For this review, take the finished solid that the model builds, in its own axes (mm). Coordinates: 2 decimals unless noted, no trailing zeros. Loops run counter-clockwise (first coordinate to the right, second up) from the corner with the lowest first, then second, coordinate; pieces in that order, holes last.
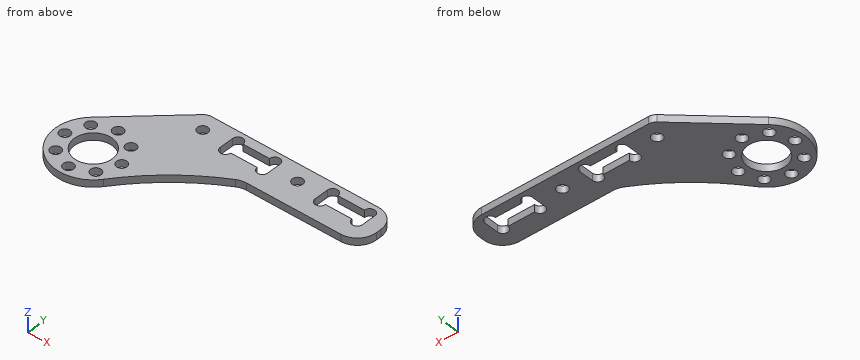
Autodesk Inventor part; units mm, degrees
ref_plane "YZ Plane" through (0, 0, 0) normal (1, 0, 0) x (0, 1, 0)
ref_plane "XZ Plane" through (0, 0, 0) normal (0, 1, 0) x (-1, 0, 0)
ref_plane "XY Plane" through (0, 0, 0) normal (0, 0, 1) x (1, 0, 0)
sketch "スケッチ1" plane through (0, 0, 0) normal (0, 0, 1) x (1, 0, 0)
  circle A0 centre (8.8, 8.8) radius 8
  circle A1 centre (2.8, 8.8) radius 0.825
  circle A2 centre (4.5574, 4.5574) radius 0.825
  circle A3 centre (8.8, 2.8) radius 0.825
  circle A4 centre (13.0426, 4.5574) radius 0.825
  circle A5 centre (14.8, 8.8) radius 0.825
  circle A6 centre (13.0426, 13.0426) radius 0.825
  circle A7 centre (8.8, 14.8) radius 0.825
  circle A8 centre (4.5574, 13.0426) radius 0.825
  circle A9 centre (8.8, 8.8) radius 4
  circle A10 centre (8.8, 14.8) radius 1.1
  circle A11 centre (4.5574, 13.0426) radius 1.1
  circle A12 centre (2.8, 8.8) radius 1.1
  circle A13 centre (4.5574, 4.5574) radius 1.1
  circle A14 centre (8.8, 2.8) radius 1.1
  circle A15 centre (13.0426, 4.5574) radius 1.1
  circle A16 centre (14.8, 8.8) radius 1.1
  circle A17 centre (13.0426, 13.0426) radius 1.1
  line L0 (3.3206, 14.6289) -> (16.8, 27.3)
  line L1 (23.8, 25.3) -> (33.8, 25.3)
  line L2 (33.8, 25.3) -> (33.8, 22.3)
  line L3 (33.8, 22.3) -> (23.8, 22.3)
  line L4 (23.8, 22.3) -> (23.8, 25.3)
  circle A18 centre (24.9, 25.3) radius 1.1
  line L5 (28.8, 25.3) -> (28.8, 22.3) construction
  line L6 (28.8, 23.8) -> (23.8, 23.8) construction
  circle A19 centre (24.9, 22.3) radius 1.1
  circle A20 centre (32.7, 25.3) radius 1.1
  circle A21 centre (32.7, 22.3) radius 1.1
  circle A22 centre (38.8, 23.8) radius 1.1
  circle A23 centre (18.8, 23.8) radius 1.1
  line L7 (16.8, 27.3) -> (40.8, 27.3)
  line L8 (40.8, 27.3) -> (40.8, 21.8)
  arc A24 (40.8, 21.8) -> (15.1891, 3.9855) centre (55.1209, -26.1052) ccw
  point P0 (0, 0)
  point P1 (31.6, 22.3)
  point P2 (26, 22.3)
  point P3 (26, 25.3)
  point P4 (31.6, 25.3)
  dimension "d7" = 2.2
  dimension "d0" = 2.2
  dimension "d3" = 360
  dimension "d5" = 10
  dimension "d6" = 3
  dimension "d8" = 2.2
  dimension "d9" = 5
  dimension "d10" = 2
  dimension "d11" = 2
  dimension "d12" = 2
  dimension "d13" = 20
  dimension "d14" = 2
  dimension "d15" = 15
  dimension "d16" = 50
extrude "押し出し1" add sketch "スケッチ1" along normal blind 1.5 contours A0 | A0 L0 L7 L8 A24
fillet "フィレット1" radius 2 3 edges at (40.8, 27.3, 0.75) (40.8, 21.8, 0.75) (16.8, 27.3, 0.75)
sketch "スケッチ4" plane through (0, 0, 0) normal (0, 0, -1) x (-1, 0, 0)
  line L0 (-53.8, 25.3) -> (-43.8, 25.3)
  line L1 (-43.8, 25.3) -> (-43.8, 22.3)
  line L2 (-43.8, 22.3) -> (-53.8, 22.3)
  line L3 (-53.8, 22.3) -> (-53.8, 25.3)
  circle A0 centre (-38.8, 23.8) radius 1.1
  circle A1 centre (-52.7, 25.3) radius 1.1
  line L4 (-48.8, 25.3) -> (-48.8, 23.8) construction
  line L5 (-48.8, 23.8) -> (-53.8, 23.8) construction
  circle A2 centre (-44.9, 25.3) radius 1.1
  circle A3 centre (-52.7, 22.3) radius 1.1
  circle A4 centre (-44.9, 22.3) radius 1.1
  arc A5 (-15.1891, 3.9855) -> (-39.4277, 21.3682) centre (-55.1209, -26.1052) ccw
  line L6 (-31.9466, 18.2) -> (-56.8, 18.2)
  line L7 (-56.8, 18.2) -> (-56.8, 27.3)
  line L8 (-38.8, 27.3) -> (-17.5925, 27.3) construction
  line L9 (-56.8, 27.3) -> (-38.8, 27.3)
  arc A6 (-16.2226, 26.7572) -> (-17.5925, 27.3) centre (-17.5925, 25.3) ccw
  line L10 (-38.8, 27.3) -> (-17.5925, 27.3)
  arc A7 (-38.8, 27.3) -> (-40.8, 25.3) centre (-38.8, 25.3) ccw
  line L11 (-40.8, 23.2671) -> (-40.8, 25.3)
  arc A8 (-40.8, 23.2671) -> (-39.4277, 21.3682) centre (-38.8, 23.2671) ccw
  arc A9 (-15.1891, 3.9855) -> (-39.4277, 21.3682) centre (-55.1209, -26.1052) ccw construction
  arc A10 (-15.1891, 3.9855) -> (-3.3206, 14.6289) centre (-8.8, 8.8) ccw
  line L12 (-16.2226, 26.7572) -> (-3.3206, 14.6289)
  circle A11 centre (-8.8, 8.8) radius 4
  circle A12 centre (-8.8, 14.8) radius 1.1
  circle A13 centre (-4.5574, 13.0426) radius 1.1
  circle A14 centre (-2.8, 8.8) radius 1.1
  circle A15 centre (-4.5574, 4.5574) radius 1.1
  circle A16 centre (-8.8, 2.8) radius 1.1
  circle A17 centre (-13.0426, 4.5574) radius 1.1
  circle A18 centre (-14.8, 8.8) radius 1.1
  circle A19 centre (-13.0426, 13.0426) radius 1.1
  circle A20 centre (-38.8, 23.8) radius 1.1
  circle A21 centre (-18.8, 23.8) radius 1.1
  line L13 (-33.8, 25.3) -> (-33.8, 22.3)
  arc A22 (-31.6, 25.3) -> (-33.8, 25.3) centre (-32.7, 25.3) ccw
  line L14 (-26, 25.3) -> (-31.6, 25.3)
  arc A23 (-23.8, 25.3) -> (-26, 25.3) centre (-24.9, 25.3) ccw
  line L15 (-23.8, 22.3) -> (-23.8, 25.3)
  arc A24 (-26, 22.3) -> (-23.8, 22.3) centre (-24.9, 22.3) ccw
  line L16 (-31.6, 22.3) -> (-26, 22.3)
  arc A25 (-33.8, 22.3) -> (-31.6, 22.3) centre (-32.7, 22.3) ccw
  point P0 (0, 0)
  point P1 (-43.8, 23.8)
  point P2 (-39.4277, 21.3682)
  point P3 (-46, 22.3)
  point P4 (-51.6, 22.3)
  point P5 (-51.6, 25.3)
  point P6 (-46, 25.3)
  dimension "d32" = 2.2
  dimension "d30" = 10
  dimension "d31" = 5
  dimension "d33" = 3
  dimension "d34" = 3
extrude "押し出し4" add sketch "スケッチ4" against normal up to surface (1.5 mm away) contours L6 L7 L9 A7 L11 A8 A5
fillet "フィレット4" radius 4 3 edges at (56.8, 18.2, 0.75) (56.8, 27.3, 0.75) (31.9466, 18.2, 0.75)
properties part number "tesaki_new" material "アルミニウム 2014-T4"
Q1. Consider section B-B (y = 6.75). State the section outline as (x, z) points.
Q2. Consider section A-A (x = 44.9). State the section outline as (y, z) points.
Q3. Consider section C-C (x = 22). State the section outline as (y, z) points.
Q4. For pin 1 Ø3 at (x, y) = (18, 23.5) entering from -Z; pin 2 Ø0.8 at (y, z) = (24, 1) entering from +X, all flat-tipped, find the tip position at first contact; note any pin that passes through.
Q5. Wall thickness on probe 1 along Y at (x, z) = (8.8, 1); probe 2 along X at (y, z) = (23, 1.35); probe 3 along X at (y, z) = (3.75, 1.4): over which ranges is each line inside the solid? List them lowest first.
Q6. Consider section D-D (z = 0.7). Count the separate pieces of the cut face and the enclosed holes in it, then the cut area to 3 significant figures.
Model answer:
1. outline: (1.07, 0) - (5.37, 0) - (5.37, 1.5) - (1.07, 1.5) - close; (12.23, 0) - (17.43, 0) - (17.43, 1.5) - (12.23, 1.5) - close
2. outline: (18.2, 0) - (21.2, 0) - (21.2, 1.5) - (18.2, 1.5) - close; (26.4, 0) - (27.3, 0) - (27.3, 1.5) - (26.4, 1.5) - close
3. outline: (11.35, 0) - (27.3, 0) - (27.3, 1.5) - (11.35, 1.5) - close
4. pin 1: stops at z = 0
4. pin 2: stops at x = 56.79
5. probe 1: y = 0.8 to 1.7, 3.9 to 4.8, 12.8 to 13.7, 15.9 to 19.78
5. probe 2: x = 12.23 to 18.05, 19.55 to 23.8, 33.8 to 38.05, 39.55 to 43.8, 53.8 to 56.8
5. probe 3: x = 2.6 to 3.81, 5.3 to 8.25, 9.35 to 12.3, 13.79 to 15
6. separate pieces: 1
6. enclosed holes: 13
6. area: 549 mm2
